Geometry check sheet. Reference: the model listing, model coordinates, mm. A direction names the side the tool comes from. Give positions to 0.01 mm unless a question says otherwise; leave off trailing zeros. Loops run counter-clockwise (first coordinate to the right, second up) from the corner with the lowest first, then second, coordinate; pieces in that order, holes last. Notation, with made-up numbers: (-10.5, 38.5) -> (0.5, 38.5) arc R17 ccw to (0.5, 52.5) -> close; hole circle Ø5 at (63.5, 35). An arc over 180 degrees is marked (long way). Answer as a JSON object with one key per item and string values.
from build123d import *

# Parameters (mm, degrees)
SKETCH1_R           = 72.55
SKETCH1_R_2         = 4.7625
BOSS_EXTRUDE1_DEPTH = 6.35
SKETCH2_R           = 82.55
CUT_EXTRUDE1_DEPTH  = 4
SKETCH3_R           = 8.5
CUT_EXTRUDE2_DEPTH  = 3


with BuildPart() as part:
    # Sketch1 → Boss-Extrude1 (new body)
    with BuildSketch(Plane.XY):
        with BuildLine():
            Line((-75, -95), (75, -95))
            ThreePointArc((75, -95), (89.142135624, -89.142135624), (95, -75))
            Line((95, -75), (95, 75))
            ThreePointArc((95, 75), (89.142135624, 89.142135624), (75, 95))
            Line((75, 95), (-75, 95))
            ThreePointArc((-75, 95), (-89.142135624, 89.142135624), (-95, 75))
            Line((-95, 75), (-95, -75))
            ThreePointArc((-95, -75), (-89.142135624, -89.142135624), (-75, -95))
        make_face()
        Circle(SKETCH1_R, mode=Mode.SUBTRACT)
        with Locations((-75, 75)):
            Circle(SKETCH1_R_2, mode=Mode.SUBTRACT)
        with Locations((75, 75)):
            Circle(SKETCH1_R_2, mode=Mode.SUBTRACT)
        with Locations((75, -75)):
            Circle(SKETCH1_R_2, mode=Mode.SUBTRACT)
        with Locations((-75, -75)):
            Circle(SKETCH1_R_2, mode=Mode.SUBTRACT)
    extrude(amount=BOSS_EXTRUDE1_DEPTH)

    # Sketch2 → Cut-Extrude1 (cut)
    with BuildSketch(Plane.XY.offset(6.35)):
        Circle(SKETCH2_R)
    extrude(amount=-CUT_EXTRUDE1_DEPTH, mode=Mode.SUBTRACT)

    # Sketch3 → Cut-Extrude2 (cut)
    with BuildSketch(Plane(origin=(0, 0, 0), x_dir=(-1, 0, 0), z_dir=(0, 0, -1))):
        with Locations((-75, 75)):
            Circle(SKETCH3_R)
        with Locations((75, 75)):
            Circle(SKETCH3_R)
        with Locations((75, -75)):
            Circle(SKETCH3_R)
        with Locations((-75, -75)):
            Circle(SKETCH3_R)
    extrude(amount=-CUT_EXTRUDE2_DEPTH, mode=Mode.SUBTRACT)


solid = part.part
1) Draft check along Y on faces 4 (the face through (83.49, 75.37, 1.48)), 5 (the face through (-65, 44, 0)), 6 (the face through (-66.51, -74.63, 1.48)), 7 (the face through (1, 95, 3)). Enter one of: pulls with the +Y half, pulls with the -Y half, needs draft (parallel to the pull), parting line crosses it, or undercut.
Geometry check:
{"face 4": "undercut", "face 5": "needs draft", "face 6": "undercut", "face 7": "pulls with the +Y half"}
2) Section check A-A on z = 1. Record the cut outline in (x, y), plus the area to 3 significant figures.
Geometry check:
{"outline": "(-95, -75) arc R20 ccw to (-75, -95) -> (75, -95) arc R20 ccw to (95, -75) -> (95, 75) arc R20 ccw to (75, 95) -> (-75, 95) arc R20 ccw to (-95, 75) -> close; hole circle Ø17 at (-75, -75); hole circle Ø17 at (-75, 75); hole circle Ø145.1 at (0, 0); hole circle Ø17 at (75, -75); hole circle Ø17 at (75, 75)", "area": "18,300 mm2"}
3) Depth check by flat-ended pin: P1, Ø13.5, axis at x = -79, y = -79, coming from the -Z side; P2, Ø12, axis at x = -74, y = 17, coming from the +Z side; P3, Ø5, axis at x = -74, y = 78, coming from the -Z side. Enter the tip coordinate at first touch or a pass-through.
Geometry check:
{"P1": "stops at z = 0", "P2": "stops at z = 2.35", "P3": "stops at z = 3"}
4) Tool access check on faces 1 (the face through (-17.895, -80.587, 4.378)), 2 (the face through (-66.51, 75.37, 1.48)), 3 (the face through (-95, 1, 3)). Record the directions out of +Z, -Z, +X, -X, +Y, -Y that give a thin tool (end or side, any length) a straight path to the whole face; none if there is none.
Geometry check:
{"face 1": "+Z", "face 2": "-Z", "face 3": "+Z, -Z, -X, +Y, -Y"}
5) Material ranges on line 1 along Y through (x, z) = (75, 2.2); line 2 along Y through (x, z) = (-1, 2.5); line 3 along Y through (x, z) = (75, 4.75), recorded low to high. Write a range as from..to.
Geometry check:
{"line 1": "y = -95..-83.5, -66.5..66.5, 83.5..95", "line 2": "y = -95..-82.54, 82.54..95", "line 3": "y = -95..-79.76, -70.24..-34.49, 34.49..70.24, 79.76..95"}
6) Section check C-C on x = 4. Record the cut outline in (y, z), plus the area to 3 significant figures.
Geometry check:
{"outline": "(-95, 0) -> (-72.44, 0) -> (-72.44, 2.35) -> (-82.45, 2.35) -> (-82.45, 6.35) -> (-95, 6.35) -> close; (72.44, 0) -> (95, 0) -> (95, 6.35) -> (82.45, 6.35) -> (82.45, 2.35) -> (72.44, 2.35) -> close", "area": "206 mm2"}
7) Section check B-B on y = 0. Record the cut outline in (x, z).
Geometry check:
{"outline": "(-95, 0) -> (-72.55, 0) -> (-72.55, 2.35) -> (-82.55, 2.35) -> (-82.55, 6.35) -> (-95, 6.35) -> close; (72.55, 0) -> (95, 0) -> (95, 6.35) -> (82.55, 6.35) -> (82.55, 2.35) -> (72.55, 2.35) -> close"}
